```python
from build123d import *

# Parameters (mm, degrees)
SKETCH2_R           = 15
SKETCH3_R           = 5
BOSS_EXTRUDE1_DEPTH = 30
SKETCH4_R           = 10
BOSS_EXTRUDE2_DEPTH = 35


with BuildPart() as part:
    # Sweep2: sweep along a path in Sketch1
    with BuildLine(Plane(origin=(0, 0, 0), x_dir=(1, 0, 0), z_dir=(0, 1, 0))) as sweep2_path:
        Line((0, 0), (885, 0))
        ThreePointArc((885, 0), (906.213203436, -8.786796564), (915, -30))
        Line((915, -30), (915, -55))
    # Sketch2 → Sweep2 (sweep)
    with BuildSketch(Plane(origin=(0, 0, 0), x_dir=(0, 0, -1), z_dir=(1, 0, 0))):
        Circle(SKETCH2_R)
    sweep(path=sweep2_path.line)

    # Sketch3 → Boss-Extrude1 (add)
    with BuildSketch(Plane.XY.offset(55)):
        with Locations((915, 0)):
            Circle(SKETCH3_R)
    extrude(amount=BOSS_EXTRUDE1_DEPTH)

    # Sketch4 → Boss-Extrude2 (add)
    with BuildSketch(Plane.XY):
        with Locations((15, 0)):
            Circle(SKETCH4_R)
    extrude(amount=-BOSS_EXTRUDE2_DEPTH)


solid = part.part
```
Input: part model. Units: mm. Frame: model coordinates. A direction names the side the tool comes from. Round coordinates to 2 decimals unless told otherwise and drop trailing zeros. Order: outer loops, then holes, each group sorted by start corner. A loop starts at its lowest first (then second) coordinate and runs counter-clockwise, first axis right, second up. Notation, with made-up numbers: (-37.5, 50.5) - (-11.5, 50.5) arc R22 ccw to (-11.5, 57.5) - close; hole circle Ø8 at (50.25, 28.5). An arc over 180 degrees is marked (long way). One line per question, with ' | ' between items. Start each with the question number.
1) Cut plane C-C, the plane x = 15. Return the cut outline in (y, z).
2) Set-up query: faces 1 (the cylindrical face through (448.695, 0.66, 14.985)), 2 (the flat face through (0, 0, 0)), 3 (the flat face through (911, 4, 55)), 4 (the cylindrical face through (24.237, -3.83, -22.923)). Return all of +Z, -Z, +X, -X, +Y, -Y with unobstructed straight access to the full face (end or side cutting, diameter ignored); none if empty.
3) Contact query for flat-ended pins moving along their axis: P1, Ø4, axis at y = 10.5, z = 47, coming from the +X side; P2, Ø1, axis at x = 561.5, y = -2.5, coming from the +Z side; P3, Ø6, axis at y = 5, z = 64, coming from the +X side. Output: stop coordinate, or through.
4) Ray query, probe 1 along X at (y, z) = (-1, 61); probe 2 along Z at (x, y) = (46, 1.5); probe 3 along Z at (x, y) = (617.5, 1). Return the intervals inside material, ascending.
5) Cut plane A-A, the plane y = 0. Return the cut outline in (x, z), then the cut area to 3 significant figures.
6) Cut plane B-B, the plane x = 760. Return the cut outline in (y, z), then the cut area to 3 significant figures.
Worked out:
1) outline: (-10, -35) - (10, -35) - (10, -11.18) arc R15 ccw (long way) to (-10, -11.18) - close
2) face 1: none | face 2: +Z, -Z, -X, +Y, -Y | face 3: +Z | face 4: -Z
3) P1: stops at x = 927.36 | P2: stops at z = 14.87 | P3: stops at x = 919.58
4) probe 1: x = 910.1 to 919.9 | probe 2: z = -14.92 to 14.92 | probe 3: z = -14.97 to 14.97
5) outline: (0, -15) - (5, -15) - (5, -35) - (25, -35) - (25, -15) - (885, -15) arc R45 ccw to (930, 30) - (930, 55) - (920, 55) - (920, 85) - (910, 85) - (910, 55) - (900, 55) - (900, 30) arc R15 cw to (885, 15) - (0, 15) - close | area: 29,400 mm^2
6) outline: circle Ø30 at (0, 0) | area: 707 mm^2
